Can you work these out from the model? Positions are in its coordinate system, mm. A direction names the side the tool comes from. Coordinates: 2 decimals unless noted, no trailing zeros. Loops run counter-clockwise (first coordinate to the right, second up) from the corner with the lowest first, then second, coordinate; pieces in that order, holes last. Notation, with made-up numbers: (-18.5, -38) - (-8.5, -38) arc R14 ccw to (-8.5, -15) - close; hole circle Ø9 at (34.5, 5). An arc over 180 degrees is marked (long way). Put each result on its own line as item: value. Start each with the question number.
Autodesk Fusion 360 part; units mm, degrees
sketch "スケッチ1" plane through (0, 0, 0) normal (0, 0, 1) x (1, 0, 0)
  line L0 (-3.5, 163) -> (-86.5, 163)
  line L1 (-86.5, 163) -> (-86.5, -163)
  line L2 (-86.5, -163) -> (-3.5, -163)
  line L3 (86.5, 25) -> (86.5, 155)
  line L4 (82.2546, 155) -> (-86.5, -163) construction
  line L5 (-86.5, 163) -> (39.184, -73.838) construction
  line L6 (-3.5, 163) -> (-3.5, 155)
  line L7 (-3.5, 155) -> (86.5, 155)
  line L8 (-86.5, -163) -> (-3.5, -163) construction
  line L9 (86.5, 25) -> (-3.5, -163)
  dimension "d2" = 326
  dimension "d5" = 83
extrude "押し出し1" add sketch "スケッチ1" along normal blind 6
chamfer "面取り1" distance 30 angle 45 2 edges at (-86.5, -163, 3) (-86.5, 163, 3)
sketch "スケッチ2" plane through (0, 0, 6) normal (0, 0, 1) x (-1, 0, 0)
  line L0 (56.5, -163) -> (86.5, -133)
  line L1 (86.5, -133) -> (86.5, 133)
  line L2 (86.5, 133) -> (56.5, 163)
  line L3 (56.5, 163) -> (3.5, 163)
  line L4 (3.5, 163) -> (-86.5, -25)
  line L5 (-86.5, -25) -> (-86.5, -155)
  line L6 (-86.5, -155) -> (3.5, -155)
  line L7 (3.5, -155) -> (3.5, -163)
  line L8 (3.5, -163) -> (56.5, -163)
  line L9 (-86.5, -155) -> (-46.5, -155) construction
  line L10 (-46.5, -155) -> (-46.5, -125) construction
  line L11 (-46.5, -125) -> (-86.5, -125) construction
  line L12 (-86.5, -125) -> (-86.5, -155) construction
  line L13 (-46.5, -125) -> (-46.5, -75) construction
  point P0 (-46.5, -125)
  point P1 (-46.5, -75)
  dimension "d10" = 40
  dimension "d11" = 30
  dimension "d12" = 50
hole "穴1" at (46.5, 125, 6) at (46.5, 75, 6) direction (0, 0, -1) diameter 18 end through all
equation "d5 = 30 mm + 53 mm"
Q1. I want a section at C-C on x = 46.5. List the corners of the cut face in (y, z) for me.
Q2. I want a section at D-D on x = -69. List the corners of the cut face in (y, z) for me.
Q3. We'd pull the mould along Y, two halves only. Please class faces 3 (the cylindrical face through (38.91, 120.16, 2.96)), 4 (the flat face through (41, 155, 3)), 5 (the flat face through (-71.7, -147.8, 3)): released by +Y, released by -Y, zero draft, split by the parting line, or undercut.
Q4. On a 3-axis mill with a long thin cutter (end or side, diameter ignored), from which of +Z, -Z, +X, -X, +Y, -Y can I reach the whole of each face in a straight line? I mean faces 1 (the flat face through (-71.3, 148.2, 3)), 2 (the flat face through (-3.5, 159, 3)). Say none if no direction works.
Q5. I want a section at B-B on z = 1.8. List the corners of the cut face in (x, y) for me.
Q6. I want a section at A-A on y = 75. List the corners of the cut face in (x, z) for me.
Q7. Please list where these lines run through material, in increasing order: line 1 along X through (y, z) = (125, 3.35); line 2 along Y through (x, z) = (42, 4.7); line 3 along Y through (x, z) = (46.5, 4.8). Write a range as [from, to].
Q8. Will this pin go through, and if not, where does the flat tip stop? pin 1 (3 mm diameter, centred on y = 157.5, z = 2.5, fed in from +X).
Calculated:
1. outline: (-58.56, 0) - (66, 0) - (66, 6) - (-58.56, 6) - close; (84, 0) - (116, 0) - (116, 6) - (84, 6) - close; (134, 0) - (155, 0) - (155, 6) - (134, 6) - close
2. outline: (-150.5, 0) - (150.5, 0) - (150.5, 6) - (-150.5, 6) - close
3. face 3: undercut
3. face 4: released by +Y
3. face 5: released by -Y
4. face 1: +Z, -Z, -X, +Y
4. face 2: +Z, -Z, +X, +Y
5. outline: (-86.5, -133) - (-56.5, -163) - (-3.5, -163) - (86.5, 25) - (86.5, 155) - (-3.5, 155) - (-3.5, 163) - (-56.5, 163) - (-86.5, 133) - close; hole circle Ø18 at (46.5, 75); hole circle Ø18 at (46.5, 125)
6. outline: (-86.5, 0) - (37.5, 0) - (37.5, 6) - (-86.5, 6) - close; (55.5, 0) - (86.5, 0) - (86.5, 6) - (55.5, 6) - close
7. line 1: [-86.5, 37.5], [55.5, 86.5]
7. line 2: [-67.96, 67.21], [82.79, 117.21], [132.79, 155]
7. line 3: [-58.56, 66], [84, 116], [134, 155]
8. pin 1: x = -3.5
